from build123d import *

# Parameters (mm, degrees)
F0_R     = 12.189783
F0_R_2   = 8.77531
F1_DEPTH = 25.4
F2_R     = 5.126436
F2_R_2   = 5.449077
F3_DEPTH = 12.7
F4_R     = 4.664571
F4_R_2   = 5.13789
F5_DEPTH = 12.7


with BuildPart() as f1:
    # F0 (on Front) → F1 (new body)
    with BuildSketch(Plane.XZ):
        Circle(F0_R)
        Circle(F0_R_2, mode=Mode.SUBTRACT)
    extrude(amount=F1_DEPTH)

    # F2 (on Front) → F3 (join)
    with BuildSketch(Plane.XZ):
        with BuildLine():
            Line((-12.411189, 60.850978), (-12.411189, 0))
            ThreePointArc((-12.411189, 0), (0, -12.411189), (12.411188, 0))
            Line((12.411188, 0), (12.411188, 60.850978))
            ThreePointArc((12.411188, 60.850978), (0, 73.262167), (-12.411189, 60.850978))
        make_face()
        Circle(F2_R, mode=Mode.SUBTRACT)
        with Locations((0, 60.850978)):
            Circle(F2_R_2, mode=Mode.SUBTRACT)
    extrude(amount=-F3_DEPTH)

    # F4 (on face) → F5 (join)
    with BuildSketch(Plane.XZ.offset(25.4)):
        with BuildLine():
            Line((-12.189783, 60.994357), (-12.189783, 0))
            ThreePointArc((-12.189783, 0), (0, -12.189783), (12.189783, 0))
            Line((12.189783, 0), (12.189783, 60.994357))
            ThreePointArc((12.189783, 60.994357), (0, 73.18414), (-12.189783, 60.994357))
        make_face()
        Circle(F4_R, mode=Mode.SUBTRACT)
        with Locations((0, 60.994357)):
            Circle(F4_R_2, mode=Mode.SUBTRACT)
    extrude(amount=F5_DEPTH)


solid = f1.part
The listing builds one solid part. Answer for the finished solid, in the listing's coordinates (mm). A direction names the side the tool comes from. Give positions to 0.01 mm unless a question says otherwise; leave off trailing zeros. Write each loop counter-clockwise with the first axis right and the second up, starting at its lowest first coordinate (ties: lowest second). Pieces come first, ordered by that corner, then holes. Notation, with made-up numbers: (3, -21) -> (48, -21) arc R36 cw to (48, 15) -> close; hole circle Ø4 at (-39.5, -29.5). An arc over 180 degrees is marked (long way). Use a Markdown table: item, result.
(1) Section B-B, the plane x = 0 is taken. Give the number of separate pieces and of enclosed holes in the cut face, then the cut area to 3 significant figures.
Return value:
| item | result |
|---|---|
| separate pieces | 4 |
| enclosed holes | 0 |
| area | 1,830 mm2 |
(2) For faces 1 (the flat face through (4, -25.4, -4)), 2 (the flat face through (-12.19, -32, 31)), 3 (the cylindrical face through (0.27, -31.66, 73.18)), 4 (the flat face through (12.19, -32, 30)), determine the directions among +Z, -Z, +X, -X, +Y, -Y from which every point of the face is accessible in a straight line to the end or side of a thin tool.
Return value:
| item | result |
|---|---|
| face 1 | none |
| face 2 | +Z, -Z, -X, -Y |
| face 3 | +Z, -Y |
| face 4 | +Z, -Z, +X, -Y |
(3) Find the intervals of material crossed by probe 1 along Z at (x, y) = (0, 5.5); probe 2 along Y at (x, z) = (-10.5, 58); probe 3 along Z at (x, y) = (0, -13.5), in increasing order. Write a range as from..to.
Return value:
| item | result |
|---|---|
| probe 1 | -12.41..-5.13, 5.13..55.4, 66.3..73.26 |
| probe 2 | -38.1..-25.4, 0..12.7 |
| probe 3 | -12.19..-8.78, 8.78..12.19 |
(4) Flat-ended cylindrical pins translate along their axes: P1, Ø4, axis at y = -4, z = 11.5, coming from the +X side; P2, Ø8, axis at x = 2.5, y = -27.5, coming from the +Z side; P3, Ø3, axis at x = -8.5, y = -15.5, coming from the +Z side. Find the tip coordinate at first contact, or state that the pin passes through.
Return value:
| item | result |
|---|---|
| P1 | x = 7.64 |
| P2 | z = 73.18 |
| P3 | z = 9.98 |
(5) Section A-A, the plane z = 36 is taken. Determine the outline of the cut face in (x, y), then the cut area to 3 significant figures.
Return value:
| item | result |
|---|---|
| outline | (-12.41, 0) -> (12.41, 0) -> (12.41, 12.7) -> (-12.41, 12.7) -> close; (-12.19, -38.1) -> (12.19, -38.1) -> (12.19, -25.4) -> (-12.19, -25.4) -> close |
| area | 625 mm2 |
(6) Section D-D, the plane x = 9.75 is taken. Determine the outline of the cut face in (y, z), then the cut area to 3 significant figures.
Return value:
| item | result |
|---|---|
| outline | (-38.1, -7.32) -> (0, -7.32) -> (0, -7.68) -> (12.7, -7.68) -> (12.7, 68.53) -> (0, 68.53) -> (0, 7.32) -> (-25.4, 7.32) -> (-25.4, 68.31) -> (-38.1, 68.31) -> close |
| area | 2,300 mm2 |
(7) Determine the mould class of faces 5 (the flat face through (-12.411, 6, 31)), 6 (the cylindrical face through (-4.07, 6.26, -3.12)), 7 (the cylindrical face through (8.106, -12.522, -3.361)), 8 (the flat face through (0, -25.4, 37)) for opening direction X: released by +X, released by -X, zero draft, split by the parting line, or undercut.
Return value:
| item | result |
|---|---|
| face 5 | released by -X |
| face 6 | undercut |
| face 7 | undercut |
| face 8 | zero draft |
(8) Section C-C, the plane y = 7 is taken. Determine the outline of the cut face in (x, z), then the cut area to 3 significant figures.
Return value:
| item | result |
|---|---|
| outline | (-12.41, 0) arc R12.41 ccw to (12.41, 0) -> (12.41, 60.85) arc R12.41 ccw to (-12.41, 60.85) -> close; hole circle Ø10.9 at (0, 60.85); hole circle Ø10.25 at (0, 0) |
| area | 1,820 mm2 |
